Source: CAD feature listing. Evaluate the final solid. Frame: model axes, mm. Round coordinates to 2 decimals unless told otherwise and drop trailing zeros. Order: outer loops, then holes, each group sorted by start corner. A loop starts at its lowest first (then second) coordinate and runs counter-clockwise, first axis right, second up.
```python
from build123d import *

# Parameters (mm, degrees)
F1_ANGLE       = 90
F2_W           = 40
F2_H           = 50
F3_ANGLE_BACK  = 5
F3_ANGLE       = 5
F4_W           = 40
F4_H           = 50
F5_ANGLE_START = 355
F5_ANGLE       = 5


with BuildPart() as f1:
    # F0 (on Front) → F1 (revolve)
    with BuildSketch(Plane.XZ):
        with BuildLine():
            Line((32, 25), (-8, 25))
            Line((-8, 25), (-8, 12.6885775404))
            ThreePointArc((-8, 12.6885775404), (15, 0), (-8, -12.6885775404))
            Line((-8, -12.6885775404), (-8, -25))
            Line((-8, -25), (32, -25))
            Line((32, -25), (32, 25))
        make_face()
    revolve(axis=Axis((-245, 0, -6.2683299184), (0, 0, -1)), revolution_arc=F1_ANGLE)

    # F2 (on face) → F3 (revolve)
    with BuildSketch(Plane(origin=(0, 0, 0), x_dir=(-1, 0, 0), z_dir=(0, 1, 0)), mode=Mode.PRIVATE) as f3_sk:
        with Locations((-12, 0)):
            Rectangle(F2_W, F2_H)
    revolve(f3_sk.sketch.rotate(Axis((-245, 0, 3.9664339274), (0, 0, 1)), -F3_ANGLE_BACK), axis=Axis((-245, 0, 3.9664339274), (0, 0, 1)), revolution_arc=F3_ANGLE)

    # F4 (on face) → F5 (revolve)
    with BuildSketch(Plane(origin=(-245, 0, 0), x_dir=(0, -1, 0), z_dir=(-1, 0, 0)), mode=Mode.PRIVATE) as f5_sk:
        with Locations((257, 0)):
            Rectangle(F4_W, F4_H)
    revolve(f5_sk.sketch.rotate(Axis((-245, 0, -1.3688886538), (0, 0, -1)), F5_ANGLE_START), axis=Axis((-245, 0, -1.3688886538), (0, 0, -1)), revolution_arc=F5_ANGLE)


solid = f1.part
```
1. Line query: line 1 along Z through (x, y) = (-49, -159.5); line 2 along Z through (x, y) = (-88, -195); line 3 along Y through (x, z) = (-63, -23). Output: solid intervals per line, ascending.
2. First-contact query: pin 1 (10 mm diameter, centred on x = -71, z = 2.5, fed in from +Y); pin 2 (2 mm diameter, centred on y = -199.5, z = 14.5, fed in from -X); pin 3 (5 mm diameter, centred on x = -119, z = 1, fed in from -Y). Flat tips, straight axial feed; report the tip coordinate or a pass-through.
3. Section A-A on z = 3. Return loops of the section in (x, y).
4. Pull-direction query (Y, two-part tool) for faces 1 (the face through (2.71, -21.67, 0.21)), 2 (the face through (-76, -170, 25)), 3 (the face through (12, 0, 0)); classes: released by +Y, released by -Y, zero draft, split by the parting line, or undercut.
Result:
1. line 1: z = -25 to -12.87, 12.87 to 25
1. line 2: z = -25 to -14.01, 14.01 to 25
1. line 3: y = -208.82 to -151.81
2. pin 1: stops at y = -188.01
2. pin 2: stops at x = -118.63
2. pin 3: stops at y = -247.95
3. outline: (-245, -277) arc R277 ccw to (32, 0) - (-8, 0) arc R237 cw to (-8.9, -20.66) - (13.71, -22.63) arc R259.7 cw to (-222.37, -258.71) - (-224.34, -236.1) arc R237 cw to (-245, -237) - close
4. face 1: undercut
4. face 2: zero draft
4. face 3: released by +Y
